```python
from build123d import *

# Parameters (mm, degrees)
SKIZZE1_R                       = 10
SKIZZE1_R_2                     = 1.5
AUFSATZ_LINEAR_AUSTRAGEN1_DEPTH = 8
SKIZZE2_W                       = 4
SKIZZE2_H                       = 22.736350236
SCHNITT_LINEAR_AUSTRAGEN1_DEPTH = 3
SKIZZE3_R                       = 3.5
SCHNITT_LINEAR_AUSTRAGEN2_DEPTH = 3


with BuildPart() as part:
    # Skizze1 → Aufsatz-Linear austragen1 (new body)
    with BuildSketch(Plane(origin=(0, 0, 0), x_dir=(1, 0, 0), z_dir=(0, 1, 0))):
        Circle(SKIZZE1_R)
        with Locations((4.949747468, 4.949747468)):
            Circle(SKIZZE1_R_2, mode=Mode.SUBTRACT)
        with Locations((-4.949747468, 4.949747468)):
            Circle(SKIZZE1_R_2, mode=Mode.SUBTRACT)
        with Locations((-4.949747468, -4.949747468)):
            Circle(SKIZZE1_R_2, mode=Mode.SUBTRACT)
        with Locations((4.949747468, -4.949747468)):
            Circle(SKIZZE1_R_2, mode=Mode.SUBTRACT)
        Circle(SKIZZE1_R_2, mode=Mode.SUBTRACT)
    extrude(amount=AUFSATZ_LINEAR_AUSTRAGEN1_DEPTH)

    # Skizze2 → Schnitt-Linear austragen1 (cut)
    with BuildSketch(Plane(origin=(0, 8, 0), x_dir=(1, 0, 0), z_dir=(0, 1, 0))):
        Rectangle(SKIZZE2_W, SKIZZE2_H)
    extrude(amount=-SCHNITT_LINEAR_AUSTRAGEN1_DEPTH, mode=Mode.SUBTRACT)

    # Skizze3 → Schnitt-Linear austragen2 (cut)
    with BuildSketch(Plane.XZ):
        Circle(SKIZZE3_R)
    extrude(amount=-SCHNITT_LINEAR_AUSTRAGEN2_DEPTH, mode=Mode.SUBTRACT)


solid = part.part
```
Could you check a few things on this model? Use its own coordinates, in mm. A direction names the side the tool comes from. Round coordinates to 2 decimals unless told otherwise and drop trailing zeros. Order: outer loops, then holes, each group sorted by start corner. A loop starts at its lowest first (then second) coordinate and runs counter-clockwise, first axis right, second up. Notation, with made-up numbers: M 66,17.25 L 100,17.25 A26 cw 100,49.25 Z; hole C 67.5,-14.75 d11. An arc over 180 degrees is marked long. One line per question, with ' | ' between items. Start each with the question number.
(1) Suppose I cut it at B-B on z = 0. List the corners of the cut face in (x, y) for me.
(2) For faces 4 (the face through (-1.5, 3.99, -0.07)), 5 (the face through (0, 3, -2)), 6 (the face through (-2, 7, 0)), which set-ups out of +Z, -Z, +X, -X, +Y, -Y let a thin tool reach every point of the face, with its end or its side?
(3) Thinking about a two-plate mould opening in X: for faces 1 (the face through (-2.17, 3.94, 9.76)), 2 (the face through (2, 7, 0)), 3 (the face through (0, 0, 4)), which applies, +X half, -X half, draft (parallel to the pull), parting line (faces both ways), or undercut?
(4) Suppose I cut it at C-C on y = 6.75. List the corners of the cut face in (x, z) for me.
(5) Please list where these lines run through material, in increasing order: line 1 along Z through (x, y) = (6.25, 4.5); line 2 along X through (y, z) = (0.5, -6); line 3 along Z through (x, y) = (-5, 6.5).
(6) For P1, Ø1, axis at x = 1.5, y = 1, coming from the -Z side; P2, Ø2, axis at x = 7.5, y = 7, coming from the -Z side; P3, Ø2.5, axis at y = 7, z = -5, coming from the -X side, each with a flat end and sliding along its axis, tell me the tip position at first contact or that it passes through.
(7) Suppose I cut it at D-D on x = 4.75. List the corners of the cut face in (y, z) for me, then the cut area to 3 significant figures.
(8) Suppose I cut it at A-A on x = 0. List the corners of the cut face in (y, z) for me, then the cut area to 3 significant figures.
Geometry results:
1) outline: M -10,0 L -3.5,0 L -3.5,3 L -1.5,3 L -1.5,5 L -2,5 L -2,8 L -10,8 Z; M 1.5,3 L 3.5,3 L 3.5,0 L 10,0 L 10,8 L 2,8 L 2,5 L 1.5,5 Z
2) face 4: +Y, -Y | face 5: -Y | face 6: +Z, -Z, +Y
3) face 1: parting line | face 2: undercut | face 3: draft
4) outline: M -2,-9.8 L -2,9.8 A10 ccw Z; M 2,-9.8 A10 ccw 2,9.8 Z; hole C -4.95,-4.95 d3; hole C -4.95,4.95 d3; hole C 4.95,-4.95 d3; hole C 4.95,4.95 d3
5) line 1: -7.81 to -5.7, -4.2 to 4.2, 5.7 to 7.81 | line 2: -8 to -6.02, -3.88 to 3.88, 6.02 to 8 | line 3: -8.66 to -6.45, -3.45 to 3.45, 6.45 to 8.66
6) P1: z = -9.95 | P2: z = -7.6 | P3: x = -9.27
7) outline: M 0,-8.8 L 8,-8.8 L 8,-6.44 L 0,-6.44 Z; M 0,-3.46 L 8,-3.46 L 8,3.46 L 0,3.46 Z; M 0,6.44 L 8,6.44 L 8,8.8 L 0,8.8 Z | area: 93.2 mm²
8) outline: M 0,-10 L 5,-10 L 5,-1.5 L 3,-1.5 L 3,-3.5 L 0,-3.5 Z; M 0,3.5 L 3,3.5 L 3,1.5 L 5,1.5 L 5,10 L 0,10 Z | area: 73.0 mm²
